Design review of the part shown in the three views and the two pictorial views. Dimensions are in mm from the part's minimum x, y and z. A direction names the side the tool comes from. Coordinates: 2 decimals unless noted, no trailing zeros. Order: outer loops, then holes, each group sorted by start corner. A loop starts at its lowest first (then second) coordinate and runs counter-clockwise, first axis right, second up. Notation, with made-up numbers: (33, 75) - (48, 75) arc R21 ccw to (48, 104) - close; hole circle Ø7 at (68, -26.5). An arc over 180 degrees is marked (long way). One line per item, written item: value. Start each with the question number.
(1) To check wall thickness, follow line 1 along X through (y, z) = (3.6, 9.5) (1 decimal); line 2 along X through (y, z) = (3.9, 12) (1 decimal); line 3 along Z through (x, y) = (5.5, 3.4) (1 decimal). State the ranges of each line that lie inside material, in increasing order.
(2) Consider section B-B on y = 5. Count the separate pieces of the cut face and the enclosed holes in it.
(3) Consider section A-A on z = 10. Write out the cut boundary in (x, y) (1 decimal).
(4) Clearance check with flat-ended pins moving along their axes: pin 1 (1.1 mm diameter, centred on y = 3.5, z = 17, fed in from +X); pin 2 (5.5 mm diameter, centred on x = 12.192, z = 9.625, fed in from +Y). State where each tip first meets the part, or that it passes through.
(5) Mouldability with a two-part tool opening along Z and no side actions: class the marked faces 4, 5 and 6 as released by +Z, released by -Z, zero draft, split by the parting line, or undercut.
(6) For the marked faces 1, 2 and 3, list the 3-axis set-ups (+Z, -Z, +X, -X, +Y, -Y) from which the entire face can be reached by the end or side of a thin tool; tool diameter is ignored.
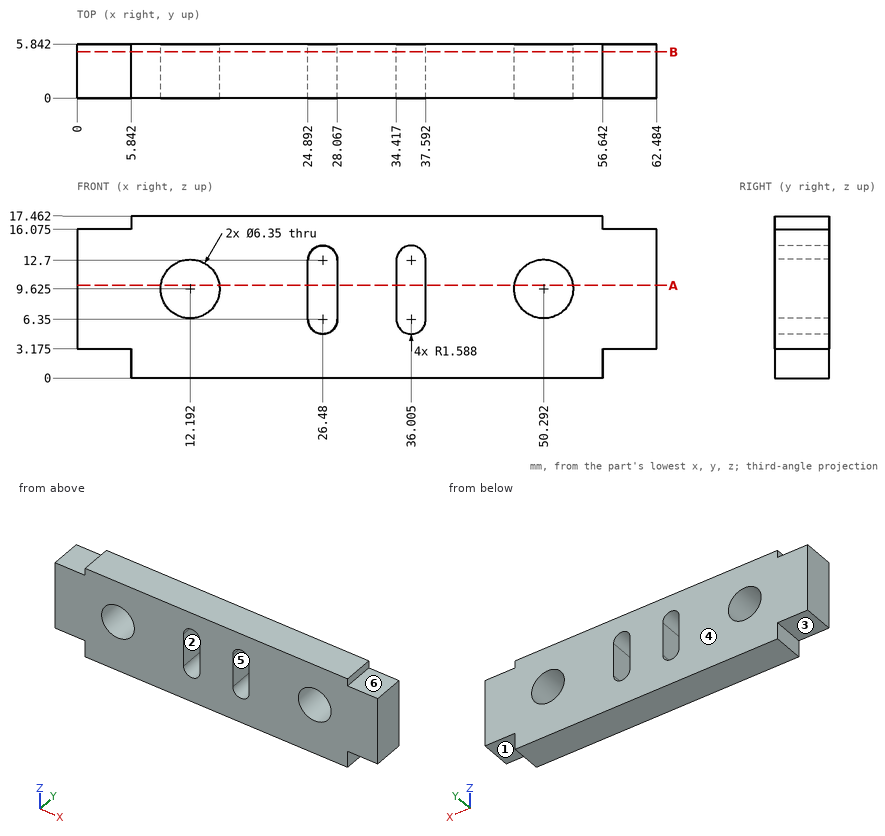
Geometry check:
1. line 1: x = 0 to 9, 15.4 to 24.9, 28.1 to 34.4, 37.6 to 47.1, 53.5 to 62.5
1. line 2: x = 0 to 10.1, 14.3 to 24.9, 28.1 to 34.4, 37.6 to 48.2, 52.4 to 62.5
1. line 3: z = 3.2 to 16.1
2. separate pieces: 1
2. enclosed holes: 4
3. outline: (0, 0) - (9, 0) - (9, 5.8) - (0, 5.8) - close; (15.3, 0) - (24.9, 0) - (24.9, 5.8) - (15.3, 5.8) - close; (28.1, 0) - (34.4, 0) - (34.4, 5.8) - (28.1, 5.8) - close; (37.6, 0) - (47.1, 0) - (47.1, 5.8) - (37.6, 5.8) - close; (53.4, 0) - (62.5, 0) - (62.5, 5.8) - (53.4, 5.8) - close
4. pin 1: stops at x = 56.64
4. pin 2: passes through
5. face 4: zero draft
5. face 5: undercut
5. face 6: released by +Z
6. face 1: -Z, +X, +Y, -Y
6. face 2: +Y, -Y
6. face 3: -Z, -X, +Y, -Y
